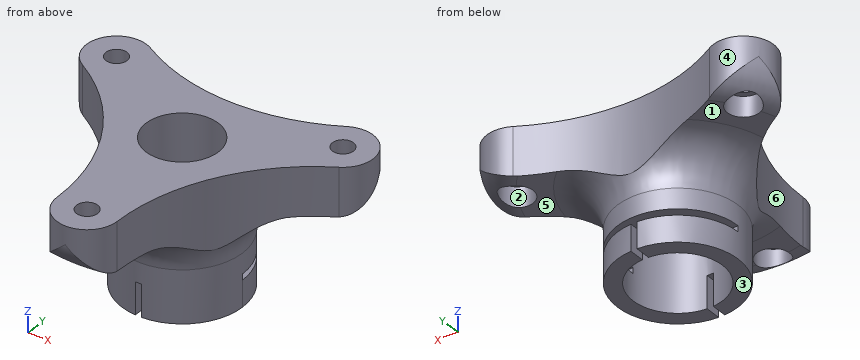
```python
from build123d import *

# Parameters (mm, degrees)
SKETCH2_R          = 11.1125
CUT_EXTRUDE1_DEPTH = 15.875
SKETCH3_W          = 35
SKETCH3_H          = 1.5
CUT_EXTRUDE2_DEPTH = 15.875
SKETCH4_W          = 1.5
SKETCH4_H          = 35
CUT_EXTRUDE3_DEPTH = 8
SKETCH8_OUTSIDE_W  = 105.686
SKETCH8_OUTSIDE_H  = 105.686
CUT_EXTRUDE4_DEPTH = 36
SKETCH9_R          = 9
CUT_EXTRUDE5_DEPTH = 20.1250001
SKETCH5_R          = 2.625
CUT_EXTRUDE7_DEPTH = 36
SKETCH11_R         = 4
CUT_EXTRUDE8_DEPTH = 5


with BuildPart() as part:
    # Sketch1 → Revolve1 (revolve)
    with BuildSketch(Plane(origin=(0, 0, 0), x_dir=(1, 0, 0), z_dir=(0, 1, 0))):
        with BuildLine():
            Line((0, 0), (40, 0))
            Line((40, 0), (40, 4.5))
            ThreePointArc((40, 4.5), (37.803300859, 9.803300859), (32.5, 12))
            Line((32.5, 12), (25, 12))
            ThreePointArc((25, 12), (17.928932188, 14.928932188), (15, 22))
            Line((15, 22), (15, 35))
            Line((15, 35), (0, 35))
            Line((0, 35), (0, 0))
        make_face()
    revolve(axis=Axis((0, 0, 0), (0, 0, -1)))

    # Sketch2 → Cut-Extrude1 (cut)
    with BuildSketch(Plane(origin=(0, 0, -35), x_dir=(-1, 0, 0), z_dir=(0, 0, -1))):
        Circle(SKETCH2_R)
    extrude(amount=-CUT_EXTRUDE1_DEPTH, mode=Mode.SUBTRACT)

    # Sketch3 → Cut-Extrude2 (cut)
    with BuildSketch(Plane(origin=(0, 0, 0), x_dir=(1, 0, 0), z_dir=(0, 1, 0))):
        with Locations((0, 27.75)):
            Rectangle(SKETCH3_W, SKETCH3_H)
    extrude(amount=CUT_EXTRUDE2_DEPTH, mode=Mode.SUBTRACT)

    # Sketch4 → Cut-Extrude3 (cut)
    with BuildSketch(Plane(origin=(0, 0, -35), x_dir=(-1, 0, 0), z_dir=(0, 0, -1))):
        Rectangle(SKETCH4_W, SKETCH4_H)
    extrude(amount=-CUT_EXTRUDE3_DEPTH, mode=Mode.SUBTRACT)

    # Sketch8 outside → Cut-Extrude4 (cut, through all)
    with BuildSketch(Plane.XY):
        Rectangle(SKETCH8_OUTSIDE_W, SKETCH8_OUTSIDE_H)
        with BuildLine():
            ThreePointArc((-24.395825623, 22.745190528), (-34.641016151, 20), (-31.895825623, 9.754809472))
            ThreePointArc((-31.895825623, 9.754809472), (-14.036841774, -8.104174377), (-7.5, -32.5))
            ThreePointArc((-7.5, -32.5), (0, -40), (7.5, -32.5))
            ThreePointArc((7.5, -32.5), (14.036841774, -8.104174377), (31.895825623, 9.754809472))
            ThreePointArc((31.895825623, 9.754809472), (34.641016151, 20), (24.395825623, 22.745190528))
            ThreePointArc((24.395825623, 22.745190528), (0, 16.208348754), (-24.395825623, 22.745190528))
        make_face(mode=Mode.SUBTRACT)
    extrude(amount=-CUT_EXTRUDE4_DEPTH, mode=Mode.SUBTRACT)

    # Sketch9 → Cut-Extrude5 (cut, through all)
    with BuildSketch(Plane(origin=(0, 0, -19.125), x_dir=(-1, 0, 0), z_dir=(0, 0, -1))):
        Circle(SKETCH9_R)
    extrude(amount=-CUT_EXTRUDE5_DEPTH, mode=Mode.SUBTRACT)

    # Sketch5 → Cut-Extrude7 (cut, through all)
    with BuildSketch(Plane.XY):
        with Locations((-28.145825623, 16.25)):
            Circle(SKETCH5_R)
        with Locations((28.145825623, 16.25)):
            Circle(SKETCH5_R)
        with Locations((0, -32.5)):
            Circle(SKETCH5_R)
    extrude(amount=-CUT_EXTRUDE7_DEPTH, mode=Mode.SUBTRACT)

    # Sketch11 → Cut-Extrude8 (cut)
    with BuildSketch(Plane(origin=(0, 0, -12), x_dir=(-1, 0, 0), z_dir=(0, 0, -1))):
        with Locations((-28.145825623, 16.25)):
            Circle(SKETCH11_R)
        with Locations((28.145825623, 16.25)):
            Circle(SKETCH11_R)
        with Locations((0, -32.5)):
            Circle(SKETCH11_R)
    extrude(amount=-CUT_EXTRUDE8_DEPTH, mode=Mode.SUBTRACT)


solid = part.part
```
Model file for the job. Use its own axes, mm. Face numbers are marked on the shaded views. A direction names the side the tool comes from. Coordinates: 2 decimals unless noted, no trailing zeros. Loops run counter-clockwise (first coordinate to the right, second up) from the corner with the lowest first, then second, coordinate; pieces in that order, holes last. Notation, with made-up numbers: (38, -15.5) - (77, -15.5) arc R12 ccw to (77, 0.5) - close; hole circle Ø5 at (49, 58). An arc over 180 degrees is marked (long way). Write item = value, one per line. Start each with the question number.
Item 1: 3-axis set-ups, long thin cutter, end or side, ignore diameter. For the marked faces 1, 2 and 3: which of +Z, -Z, +X, -X, +Y, -Y reach the whole face in a straight line?
Item 2: Pull direction X, two halves, no side cores. Call the marked faces 4, 5 and 6: +X half, -X half, draft (parallel to the pull), parting line (faces both ways), or undercut.
Item 3: Wall check: probe 1 along Y at (x, z) = (0, -4.25) (3 decimals); probe 2 along Z at (x, y) = (3, 14.5); probe 3 along Y at (x, z) = (0, -26.75). Give the ranges that are in metal, low to high. Write a range as [from, to].
Item 4: Saw through at C-C, the plane z = -15. List the corners of the cut face in (x, y), then the cut area to 3 significant figures.
Item 5: Saw through at A-A, the plane z = -2.5. List the corners of the cut face in (x, y) (3 decimals), then the cut area to 3 significant figures.
Item 6: Drop flat-ended pins along their axis: pin 1 Ø10 at (y, z) = (17, -20.5) entering from -X; pin 2 Ø10 at (x, y) = (22.5, 11) entering from -Z; pin 3 Ø8 at (y, z) = (-5.5, -23) entering from -X; pin 4 Ø5 at (x, y) = (-28.15, 16.25) entering from +Z. Give the stop position or say it passes through.
Item 7: Saw through at D-D, the plane z = -8. List the corners of the cut face in (x, y).
Answers:
q1.face_1 = -Z, -X, +Y
q1.face_2 = -Z
q1.face_3 = -Z, +X, -X, +Y, -Y
q2.face_4 = undercut
q2.face_5 = draft
q2.face_6 = -X half
q3.probe_1 = [-40, -35.125], [-29.875, -9], [9, 16.208]
q3.probe_2 = [-35, -28.5], [-27, 0]
q3.probe_3 = [-15, -11.11], [11.11, 15]
q4.outline = (-17.65, -2.71) arc R48.79 cw to (-11.17, -13.93) arc R17.86 ccw to (11.17, -13.93) arc R48.79 cw to (17.65, -2.71) arc R17.86 ccw to (6.48, 16.64) arc R48.79 cw to (-6.48, 16.64) arc R17.86 ccw to start; hole circle Ø18 at (0, 0)
q4.area = 704 mm2
q5.outline = (-31.896, 9.755) arc R48.792 cw to (-7.5, -32.5) arc R7.5 ccw to (7.5, -32.5) arc R48.792 cw to (31.896, 9.755) arc R7.5 ccw to (24.396, 22.745) arc R48.792 cw to (-24.396, 22.745) arc R7.5 ccw to start; hole circle Ø5.25 at (-28.146, 16.25); hole circle Ø18 at (0, 0); hole circle Ø5.25 at (0, -32.5); hole circle Ø5.25 at (28.146, 16.25)
q5.area = 1,690 mm2
q6.pin_1 = -9.5
q6.pin_2 = -13.31
q6.pin_3 = -14.93
q6.pin_4 = through
q7.outline = (-35.65, 16.15) arc R7.5 ccw to (-31.9, 9.75) arc R48.79 cw to (-7.5, -32.5) arc R7.5 ccw to (-3.84, -38.94) arc R39.13 ccw to (3.84, -38.94) arc R7.5 ccw to (7.5, -32.5) arc R48.79 cw to (31.9, 9.75) arc R7.5 ccw to (35.65, 16.15) arc R39.13 ccw to (31.81, 22.79) arc R7.5 ccw to (24.4, 22.75) arc R48.79 cw to (-24.4, 22.75) arc R7.5 ccw to (-31.81, 22.79) arc R39.13 ccw to start; hole circle Ø8 at (-28.15, 16.25); hole circle Ø18 at (0, 0); hole circle Ø8 at (0, -32.5); hole circle Ø8 at (28.15, 16.25)
